Model file for the job. Use its own axes, mm. A direction names the side the tool comes from. Round coordinates to 2 decimals unless told otherwise and drop trailing zeros. Loops run counter-clockwise (first coordinate to the right, second up) from the corner with the lowest first, then second, coordinate; pieces in that order, holes last. Notation, with made-up numbers: (-3, 51) -> (17, 51) arc R6 cw to (17, 60) -> close; hole circle Ø3 at (74.25, 70). An arc over 180 degrees is marked (long way). Use a Markdown table: item, result.
from build123d import *

# Parameters (mm, degrees)
F0_R           = 25.4
F0_R_2         = 10.3251
F1_DEPTH       = 15.875
F3_D           = 4.7752
F3_CBORE_D     = 8.7376
F3_CBORE_DEPTH = 3.9624
F6_R           = 1.5875
F7_DEPTH       = 9.2980452561
F8_R           = 1.5875
F9_DEPTH       = 60.0980452561


with BuildPart() as f1:
    # F0 (on Front) → F1 (new body)
    with BuildSketch(Plane.XZ):
        Circle(F0_R)
        Circle(F0_R_2, mode=Mode.SUBTRACT)
    extrude(amount=F1_DEPTH)

    # F3 (through all)
    with Locations(Plane.XZ.offset(15.875)):
        with Locations((0, 19.05), (-16.4977839421, -9.525), (16.4977839421, -9.525)):
            CounterBoreHole(F3_D / 2, F3_CBORE_D / 2, F3_CBORE_DEPTH)

    # F6 (on face) → F7 (cut, through all)
    with BuildSketch(Plane(origin=(12.7, 0, 21.9970452561), x_dir=(0.8660254038, 0, -0.5), z_dir=(-0.5, 0, -0.8660254038))):
        with Locations((0.8242388722, 7.9502)):
            Circle(F6_R)
    extrude(amount=-F7_DEPTH, mode=Mode.SUBTRACT)

    # F8 (on face) → F9 (cut, through all)
    with BuildSketch(Plane(origin=(12.7, 0, 21.9970452561), x_dir=(0.8660254038, 0, -0.5), z_dir=(-0.5, 0, -0.8660254038))):
        with Locations((0, 7.9248)):
            Circle(F8_R)
    extrude(amount=F9_DEPTH, mode=Mode.SUBTRACT)


solid = f1.part
Q1. Band-saw the part on C-C, the plane x = -17. Give the cut face in (y, z) (3 decimals), plus the area to 3 significant figures.
Results list:
| item | result |
|---|---|
| outline | (-15.875, -18.872) -> (0, -18.872) -> (0, -11.859) -> (-11.913, -11.859) -> (-11.913, -13.865) -> (-15.875, -13.865) -> close; (-15.875, -5.185) -> (-11.913, -5.185) -> (-11.913, -7.191) -> (0, -7.191) -> (0, 18.872) -> (-15.875, 18.872) -> close |
| area | 509 mm² |
Q2. Band-saw the part on B-B, the plane z = 0. Give the cut face in (x, y) (3 decimals), plus the area to 3 significant figures.
Results list:
| item | result |
|---|---|
| outline | (-25.4, -15.875) -> (-10.325, -15.875) -> (-10.325, 0) -> (-25.4, 0) -> close; (10.325, -15.875) -> (25.4, -15.875) -> (25.4, 0) -> (10.325, 0) -> close |
| area | 479 mm² |
Q3. Tool access for faces 4 (the face through (18.4, -11.913, -11.4)), 5 (the face through (11, 0, 0)): list every direction of +Z, -Z, +X, -X, +Y, -Y with a clear straight run to the whole face (end or side of a thin tool).
Results list:
| item | result |
|---|---|
| face 4 | -Y |
| face 5 | +Z, -Z, +X, -X, +Y |
Q4. Flat gauge pins, fed straight in: pin 1 (7.5 mm diameter, centred on x = 0, z = 19.05, fed in from -Y); pin 2 (9.5 mm diameter, centred on x = -18, z = -11.5, fed in from -Y) (3 decimals); pin 3 (8 mm diameter, centred on x = 12, y = -12, fed in from +Z); pin 4 (1 mm diameter, centred on x = -11, y = -10.5, fed in from +Z). Where does each tip first touch, or does it go through?
Results list:
| item | result |
|---|---|
| pin 1 | stops at y = -11.91 |
| pin 2 | stops at y = -15.875 |
| pin 3 | stops at z = 24.11 |
| pin 4 | stops at z = 23.13 |
Q5. Band-saw the part on A-A, the plane x = 0. Give the cut face in (y, z) (3 decimals), plus the area to 3 significant figures.
Results list:
| item | result |
|---|---|
| outline | (-15.875, -25.4) -> (0, -25.4) -> (0, -10.325) -> (-15.875, -10.325) -> close; (-15.875, 10.325) -> (0, 10.325) -> (0, 16.662) -> (-11.913, 16.662) -> (-11.913, 14.681) -> (-15.875, 14.681) -> close; (-15.875, 23.419) -> (-11.913, 23.419) -> (-11.913, 21.438) -> (0, 21.438) -> (0, 25.4) -> (-15.875, 25.4) -> close |
| area | 387 mm² |
Q6. Pull direction Z, two halves, no side cores. Call faces 1 (the face through (0, -15.875, -11)), 2 (the face through (2, -11.913, 17)), 3 (the face through (-5.506, -7.826, -24.796)): released by +Z, released by -Z, zero draft, split by the parting line, or undercut.
Results list:
| item | result |
|---|---|
| face 1 | zero draft |
| face 2 | undercut |
| face 3 | split by the parting line |
Q7. Drill centre lines: L1, parallel to Z at x = 0, y = -12.9; L2, parallel to Z at x = 0, y = -8.25; L3, parallel to Y at x = -0.5, z = 16. Where is each one in solid material? Low to high. Write a range as from..to.
Results list:
| item | result |
|---|---|
| L1 | z = -25.4..-10.33, 10.33..14.68, 23.42..25.4 |
| L2 | z = -25.4..-10.33, 10.33..16.66, 21.44..25.4 |
| L3 | y = -11.91..0 |
Q8. Band-saw the part on D-D, the plane y = -1.5. Give the cut face in (x, z) (3 decimals).
Results list:
| item | result |
|---|---|
| outline | circle Ø50.8 at (0, 0); hole circle Ø4.775 at (-16.498, -9.525); hole circle Ø20.65 at (0, 0); hole circle Ø4.775 at (0, 19.05); hole circle Ø4.775 at (16.498, -9.525) |
